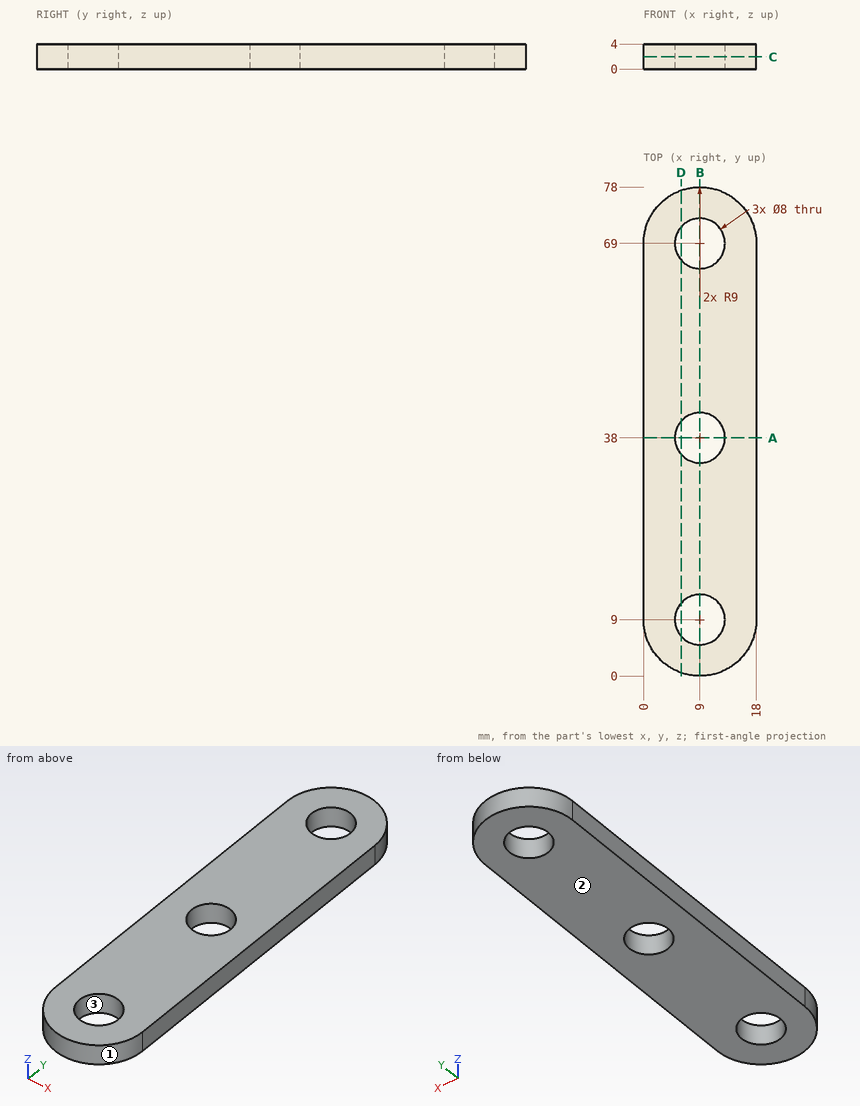
Input: dimensioned drawing with shaded views. Units: mm. Origin: part minimum x, y, z. Round coordinates to 2 decimals unless told otherwise and drop trailing zeros. Loops run counter-clockwise (first coordinate to the right, second up) from the corner with the lowest first, then second, coordinate; pieces in that order, holes last. Notation, with made-up numbers: (80.5, 68) -> (127.5, 68) arc R10 ccw to (127.5, 84) -> close; hole circle Ø1 at (2.25, 59.25). An arc over 180 degrees is marked (long way). One line per item, written item: value.
(1) Mould query, pull axis X, two halves, no side actions, for the marked faces 1, 2 and 3. Classes: pulls with the +X half, pulls with the -X half, needs draft (parallel to the pull), parting line crosses it, or undercut.
Geometry check:
face 1: parting line crosses it
face 2: needs draft
face 3: undercut
(2) Material intervals for line 1 (Y direction, x = 8.75, z = 0.4); line 2 (Y direction, x = 10.75, z = 0.25); line 3 (X direction, y = 12.5, z = 2.9), sorted ascending. Write a range as [from, to].
Geometry check:
line 1: [0, 5.01], [12.99, 34.01], [41.99, 65.01], [72.99, 78]
line 2: [0.17, 5.4], [12.6, 34.4], [41.6, 65.4], [72.6, 77.83]
line 3: [0, 7.06], [10.94, 18]
(3) Section B-B (x = 9). Return the cut outline in (y, z), plus the area to 3 significant figures.
Geometry check:
outline: (0, 0) -> (5, 0) -> (5, 4) -> (0, 4) -> close; (13, 0) -> (34, 0) -> (34, 4) -> (13, 4) -> close; (42, 0) -> (65, 0) -> (65, 4) -> (42, 4) -> close; (73, 0) -> (78, 0) -> (78, 4) -> (73, 4) -> close
area: 216 mm2
(4) Pin query (flat end, axial travel): pin 1 (1.5 mm diameter, centred on x = 11, z = 3.5, fed in from +Y); pin 2 (10.5 mm diameter, centred on x = 9, y = 69, fed in from -Z); pin 3 (2 mm diameter, centred on x = 7, z = 1.5, fed in from -Y); pin 4 (1.5 mm diameter, centred on x = 15, z = 2.5, fed in from -Y). Return the tip coordinate at first contact, or that it passes through.
Geometry check:
pin 1: y = 77.91
pin 2: z = 0
pin 3: y = 0.06
pin 4: y = 1.69
(5) Section A-A (y = 38). Return the cut outline in (x, z), plus the area to 3 significant figures.
Geometry check:
outline: (0, 0) -> (5, 0) -> (5, 4) -> (0, 4) -> close; (13, 0) -> (18, 0) -> (18, 4) -> (13, 4) -> close
area: 40.0 mm2
(6) Section C-C (z = 1.95). Return the cut outline in (x, y), plus the area to 3 significant figures.
Geometry check:
outline: (0, 9) arc R9 ccw to (18, 9) -> (18, 69) arc R9 ccw to (0, 69) -> close; hole circle Ø8 at (9, 9); hole circle Ø8 at (9, 38); hole circle Ø8 at (9, 69)
area: 1,180 mm2
(7) Section D-D (x = 6). Return the cut outline in (y, z).
Geometry check:
outline: (0.51, 0) -> (6.35, 0) -> (6.35, 4) -> (0.51, 4) -> close; (11.65, 0) -> (35.35, 0) -> (35.35, 4) -> (11.65, 4) -> close; (40.65, 0) -> (66.35, 0) -> (66.35, 4) -> (40.65, 4) -> close; (71.65, 0) -> (77.49, 0) -> (77.49, 4) -> (71.65, 4) -> close
